from build123d import *

# Parameters (mm, degrees)
SALIENTE_EXTRUIR1_DEPTH = 0.1


with BuildPart() as part:
    # Model → Saliente-Extruir1 (new body)
    with BuildSketch(Plane.XY):
        with BuildLine():
            Line((7.842607398, 33.951363828), (9.579734894, 37.856921812))
            ThreePointArc((9.579734894, 37.856921812), (5.853816343, 39.435481261), (2.446469011, 41.618209633))
            ThreePointArc((2.446469011, 41.618209633), (2.30530398, 41.73720898), (2.175714205, 41.868719058))
            ThreePointArc((2.175714205, 41.868719058), (-8.403464325, 62.063986958), (-8.03987526, 84.859505528))
            ThreePointArc((-8.03987526, 84.859505528), (1.236190849, 84.069577534), (9.603788078, 88.150350168))
            ThreePointArc((9.603788078, 88.150350168), (15.569580386, 86.351015884), (21.535340373, 88.150457325))
            ThreePointArc((21.535340373, 88.150457325), (29.9030109, 84.069834991), (39.179062819, 84.859929602))
            ThreePointArc((39.179062819, 84.859929602), (39.545951554, 62.067945489), (28.972930685, 41.873382438))
            ThreePointArc((28.972930685, 41.873382438), (28.843386689, 41.741827264), (28.702263084, 41.622778791))
            ThreePointArc((28.702263084, 41.622778791), (25.291019086, 39.436407853), (21.560299513, 37.855732375))
            Line((21.560299513, 37.855732375), (23.296856275, 33.951104051))
            ThreePointArc((23.296856275, 33.951104051), (23.379782362, 33.667159579), (23.503682681, 33.398552226))
            ThreePointArc((23.503682681, 33.398552226), (24.91201243, 35.055347002), (26.795735375, 36.141601796))
            ThreePointArc((26.795735375, 36.141601796), (27.061156988, 36.22854536), (27.331998678, 36.296755293))
            ThreePointArc((27.331998678, 36.296755293), (28.581463341, 36.797016912), (29.594274303, 37.683378907))
            ThreePointArc((29.594274303, 37.683378907), (33.634090695, 39.784233724), (37.930992822, 38.277469126))
            ThreePointArc((37.930992822, 38.277469126), (41.505714026, 35.445010711), (45.978885302, 34.554959535))
            ThreePointArc((45.978885302, 34.554959535), (46.208146888, 34.559844902), (46.437427714, 34.555966165))
            ThreePointArc((46.437427714, 34.555966165), (47.345458783, 34.798460155), (47.962246093, 35.507612586))
            ThreePointArc((47.962246093, 35.507612586), (47.867291161, 36.636427891), (47.611593039, 37.739994337))
            ThreePointArc((47.611593039, 37.739994337), (45.887992379, 43.222004619), (43.431064267, 48.416880961))
            ThreePointArc((43.431064267, 48.416880961), (41.946296228, 52.847104425), (41.234230474, 57.46493708))
            ThreePointArc((41.234230474, 57.46493708), (43.653110533, 53.102823777), (48.0017493, 50.65980227))
            ThreePointArc((48.0017493, 50.65980227), (43.593122133, 58.078880454), (42.149031339, 66.587306652))
            ThreePointArc((42.149031339, 66.587306652), (42.59469449, 68.050991275), (43.121201087, 69.487577202))
            ThreePointArc((43.121201087, 69.487577202), (46.085206987, 81.850895157), (41.113090097, 93.551964146))
            ThreePointArc((41.113090097, 93.551964146), (38.356950801, 95.965555009), (35.322319177, 98.018049973))
            ThreePointArc((35.322319177, 98.018049973), (11.172182801, 102.279245092), (-11.242648027, 92.331268928))
            ThreePointArc((-11.242648027, 92.331268928), (-14.949595702, 86.979124351), (-16.674221293, 80.701180482))
            ThreePointArc((-16.674221293, 80.701180482), (-16.531478417, 74.824409953), (-14.601116723, 69.271887003))
            ThreePointArc((-14.601116723, 69.271887003), (-12.073727961, 65.477087664), (-10.129040046, 61.353207829))
            ThreePointArc((-10.129040046, 61.353207829), (-9.555595879, 53.303802947), (-12.946389483, 45.980943128))
            ThreePointArc((-12.946389483, 45.980943128), (-15.354439926, 42.946547728), (-16.383842014, 39.212033874))
            ThreePointArc((-16.383842014, 39.212033874), (-15.350532825, 33.44879775), (-11.593101389, 28.958327007))
            ThreePointArc((-11.593101389, 28.958327007), (-9.872267141, 30.049029711), (-7.929133035, 30.661510518))
            Line((-7.929133035, 30.661510518), (-5.334790759, 30.979264145))
            ThreePointArc((-5.334790759, 30.979264145), (0.499105837, 35.811881702), (7.842607398, 33.951363828))
        make_face()
    extrude(amount=SALIENTE_EXTRUIR1_DEPTH)


solid = part.part
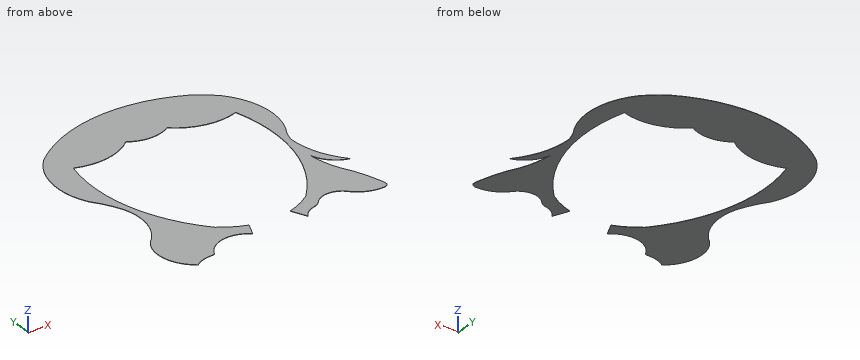
Input: part model. Units: mm. Frame: model coordinates. Coordinates: 2 decimals unless noted, no trailing zeros. Loops run counter-clockwise (first coordinate to the right, second up) from the corner with the lowest first, then second, coordinate; pieces in that order, holes last.
(1) Section B-B on y = 60. Return the cut outline in (x, z).
(2) Section C-C on y = 90. Return the cut outline in (x, z), then the cut area to 3 significant figures.
(3) Section D-D on x = 17. Return the cut outline in (y, z).
(4) Material intervals for probe 1 along Y at (x, z) = (22, 0.05); probe 2 along X at (y, z) = (68, 0.05); probe 3 along Y at (x, z) = (11, 0.05), sorted ascending.
(5) Section A-A on x = -6.5. Return the cut outline in (y, z).
Data:
1. outline: (-9.74, 0) - (-7.86, 0) - (-7.86, 0.1) - (-9.74, 0.1) - close; (39, 0) - (42.98, 0) - (42.98, 0.1) - (39, 0.1) - close
2. outline: (-13.19, 0) - (43.61, 0) - (43.61, 0.1) - (-13.19, 0.1) - close
2. area: 5.68 mm2
3. outline: (86.45, 0) - (102.58, 0) - (102.58, 0.1) - (86.45, 0.1) - close
4. probe 1: y = 36.87 to 38, 87.75 to 102.2
4. probe 2: x = -13.66 to -9.41, 40.55 to 42.58
4. probe 3: y = 87.37 to 102.26
5. outline: (30.84, 0) - (55.96, 0) - (55.96, 0.1) - (30.84, 0.1) - close; (84.37, 0) - (95.89, 0) - (95.89, 0.1) - (84.37, 0.1) - close
